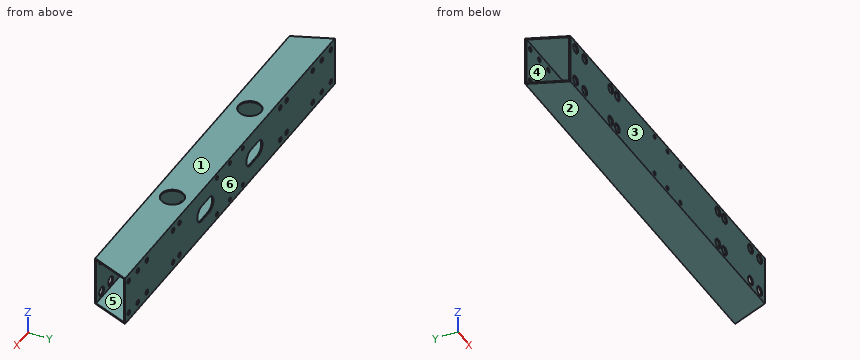
```python
from build123d import *

# Parameters (mm, degrees)
SKETCH_1_W          = 40
SKETCH_1_H          = 30
SKETCH_1_W_2        = 38
SKETCH_1_H_2        = 28
EXTRUDE_1_DEPTH     = 325
SKETCH_2_R          = 2.025
CUT_EXTRUDE_1_DEPTH = 31
SKETCH_3_R          = 2.025
CUT_EXTRUDE_2_DEPTH = 31
SKETCH_4_R          = 1.6
CUT_EXTRUDE_3_DEPTH = 31
CUT_EXTRUDE_4_DEPTH = 41
CUT_EXTRUDE_5_REACH = 32
SKETCH_6_R          = 3.75
CUT_EXTRUDE_6_REACH = 32
SKETCH_7_R          = 3.75
CUT_EXTRUDE_7_REACH = 42
SKETCH_8_R          = 9
CUT_EXTRUDE_8_REACH = 32


with BuildPart() as part:
    # 草图1 → 凸台-拉伸1 (new body)
    with BuildSketch(Plane(origin=(0, 0, 0), x_dir=(0, 0, -1), z_dir=(1, 0, 0))):
        Rectangle(SKETCH_1_W, SKETCH_1_H)
        Rectangle(SKETCH_1_W_2, SKETCH_1_H_2, mode=Mode.SUBTRACT)
    extrude(amount=EXTRUDE_1_DEPTH)

    # 草图2 → 切除-拉伸1 (cut, through all)
    with BuildSketch(Plane.XZ.offset(15)):
        with Locations((74.5, 14)):
            Circle(SKETCH_2_R)
        with Locations((84.5, 14)):
            Circle(SKETCH_2_R)
        with Locations((84.5, -14)):
            Circle(SKETCH_2_R)
        with Locations((74.5, -14)):
            Circle(SKETCH_2_R)
        with Locations((250.5, -14)):
            Circle(SKETCH_2_R)
        with Locations((240.5, -14)):
            Circle(SKETCH_2_R)
        with Locations((240.5, 14)):
            Circle(SKETCH_2_R)
        with Locations((250.5, 14)):
            Circle(SKETCH_2_R)
    extrude(amount=-CUT_EXTRUDE_1_DEPTH, mode=Mode.SUBTRACT)

    # 草图3 → 切除-拉伸2 (cut, through all)
    with BuildSketch(Plane.XZ.offset(15)):
        with Locations((291, 14)):
            Circle(SKETCH_3_R)
        with Locations((305, 14)):
            Circle(SKETCH_3_R)
        with Locations((319, 14)):
            Circle(SKETCH_3_R)
        with Locations((319, -14)):
            Circle(SKETCH_3_R)
        with Locations((305, -14)):
            Circle(SKETCH_3_R)
        with Locations((291, -14)):
            Circle(SKETCH_3_R)
        with Locations((34, -14)):
            Circle(SKETCH_3_R)
        with Locations((20, -14)):
            Circle(SKETCH_3_R)
        with Locations((6, -14)):
            Circle(SKETCH_3_R)
        with Locations((6, 14)):
            Circle(SKETCH_3_R)
        with Locations((20, 14)):
            Circle(SKETCH_3_R)
        with Locations((34, 14)):
            Circle(SKETCH_3_R)
    extrude(amount=-CUT_EXTRUDE_2_DEPTH, mode=Mode.SUBTRACT)

    # 草图4 → 切除-拉伸3 (cut, through all)
    with BuildSketch(Plane.XZ.offset(15)):
        with Locations((142.5, 16)):
            Circle(SKETCH_4_R)
        with Locations((162.5, 16)):
            Circle(SKETCH_4_R)
        with Locations((182.5, 16)):
            Circle(SKETCH_4_R)
        with Locations((182.5, -16)):
            Circle(SKETCH_4_R)
        with Locations((162.5, -16)):
            Circle(SKETCH_4_R)
        with Locations((142.5, -16)):
            Circle(SKETCH_4_R)
    extrude(amount=-CUT_EXTRUDE_3_DEPTH, mode=Mode.SUBTRACT)

    # 草图5 → 切除-拉伸4 (cut, through all)
    with BuildSketch(Plane.XY.offset(20)):
        Polygon((0, 15), (12, -15), (0, -15), align=None)
        Polygon((313, -15), (325, -15), (325, 15), align=None)
    extrude(amount=-CUT_EXTRUDE_4_DEPTH, mode=Mode.SUBTRACT)

    # 草图6 → 切除-拉伸5 (cut, up to next)
    with BuildSketch(Plane.XZ.offset(15), mode=Mode.PRIVATE) as cut_extrude_5_sk1:
        with Locations((74.5, 14)):
            Circle(SKETCH_6_R)
    cut_extrude_5_tool1 = extrude(cut_extrude_5_sk1.sketch, amount=-CUT_EXTRUDE_5_REACH, mode=Mode.PRIVATE) & part.part
    add(cut_extrude_5_tool1.solids().sort_by_distance((74.5, -15, 14))[0], mode=Mode.SUBTRACT)
    # 草图6 → 切除-拉伸5 (cut, up to next)
    with BuildSketch(Plane.XZ.offset(15), mode=Mode.PRIVATE) as cut_extrude_5_sk2:
        with Locations((84.5, 14)):
            Circle(SKETCH_6_R)
    cut_extrude_5_tool2 = extrude(cut_extrude_5_sk2.sketch, amount=-CUT_EXTRUDE_5_REACH, mode=Mode.PRIVATE) & part.part
    add(cut_extrude_5_tool2.solids().sort_by_distance((84.5, -15, 14))[0], mode=Mode.SUBTRACT)
    # 草图6 → 切除-拉伸5 (cut, up to next)
    with BuildSketch(Plane.XZ.offset(15), mode=Mode.PRIVATE) as cut_extrude_5_sk3:
        with Locations((84.5, -14)):
            Circle(SKETCH_6_R)
    cut_extrude_5_tool3 = extrude(cut_extrude_5_sk3.sketch, amount=-CUT_EXTRUDE_5_REACH, mode=Mode.PRIVATE) & part.part
    add(cut_extrude_5_tool3.solids().sort_by_distance((84.5, -15, -14))[0], mode=Mode.SUBTRACT)
    # 草图6 → 切除-拉伸5 (cut, up to next)
    with BuildSketch(Plane.XZ.offset(15), mode=Mode.PRIVATE) as cut_extrude_5_sk4:
        with Locations((74.5, -14)):
            Circle(SKETCH_6_R)
    cut_extrude_5_tool4 = extrude(cut_extrude_5_sk4.sketch, amount=-CUT_EXTRUDE_5_REACH, mode=Mode.PRIVATE) & part.part
    add(cut_extrude_5_tool4.solids().sort_by_distance((74.5, -15, -14))[0], mode=Mode.SUBTRACT)
    # 草图6 → 切除-拉伸5 (cut, up to next)
    with BuildSketch(Plane.XZ.offset(15), mode=Mode.PRIVATE) as cut_extrude_5_sk5:
        with Locations((250.5, -14)):
            Circle(SKETCH_6_R)
    cut_extrude_5_tool5 = extrude(cut_extrude_5_sk5.sketch, amount=-CUT_EXTRUDE_5_REACH, mode=Mode.PRIVATE) & part.part
    add(cut_extrude_5_tool5.solids().sort_by_distance((250.5, -15, -14))[0], mode=Mode.SUBTRACT)
    # 草图6 → 切除-拉伸5 (cut, up to next)
    with BuildSketch(Plane.XZ.offset(15), mode=Mode.PRIVATE) as cut_extrude_5_sk6:
        with Locations((240.5, -14)):
            Circle(SKETCH_6_R)
    cut_extrude_5_tool6 = extrude(cut_extrude_5_sk6.sketch, amount=-CUT_EXTRUDE_5_REACH, mode=Mode.PRIVATE) & part.part
    add(cut_extrude_5_tool6.solids().sort_by_distance((240.5, -15, -14))[0], mode=Mode.SUBTRACT)
    # 草图6 → 切除-拉伸5 (cut, up to next)
    with BuildSketch(Plane.XZ.offset(15), mode=Mode.PRIVATE) as cut_extrude_5_sk7:
        with Locations((240.5, 14)):
            Circle(SKETCH_6_R)
    cut_extrude_5_tool7 = extrude(cut_extrude_5_sk7.sketch, amount=-CUT_EXTRUDE_5_REACH, mode=Mode.PRIVATE) & part.part
    add(cut_extrude_5_tool7.solids().sort_by_distance((240.5, -15, 14))[0], mode=Mode.SUBTRACT)
    # 草图6 → 切除-拉伸5 (cut, up to next)
    with BuildSketch(Plane.XZ.offset(15), mode=Mode.PRIVATE) as cut_extrude_5_sk8:
        with Locations((250.5, 14)):
            Circle(SKETCH_6_R)
    cut_extrude_5_tool8 = extrude(cut_extrude_5_sk8.sketch, amount=-CUT_EXTRUDE_5_REACH, mode=Mode.PRIVATE) & part.part
    add(cut_extrude_5_tool8.solids().sort_by_distance((250.5, -15, 14))[0], mode=Mode.SUBTRACT)

    # 草图7 → 切除-拉伸6 (cut, up to next)
    with BuildSketch(Plane.XZ.offset(15), mode=Mode.PRIVATE) as cut_extrude_6_sk1:
        with Locations((20, 14)):
            Circle(SKETCH_7_R)
    cut_extrude_6_tool1 = extrude(cut_extrude_6_sk1.sketch, amount=-CUT_EXTRUDE_6_REACH, mode=Mode.PRIVATE) & part.part
    add(cut_extrude_6_tool1.solids().sort_by_distance((20, -15, 14))[0], mode=Mode.SUBTRACT)
    # 草图7 → 切除-拉伸6 (cut, up to next)
    with BuildSketch(Plane.XZ.offset(15), mode=Mode.PRIVATE) as cut_extrude_6_sk2:
        with Locations((34, 14)):
            Circle(SKETCH_7_R)
    cut_extrude_6_tool2 = extrude(cut_extrude_6_sk2.sketch, amount=-CUT_EXTRUDE_6_REACH, mode=Mode.PRIVATE) & part.part
    add(cut_extrude_6_tool2.solids().sort_by_distance((34, -15, 14))[0], mode=Mode.SUBTRACT)
    # 草图7 → 切除-拉伸6 (cut, up to next)
    with BuildSketch(Plane.XZ.offset(15), mode=Mode.PRIVATE) as cut_extrude_6_sk3:
        with Locations((34, -14)):
            Circle(SKETCH_7_R)
    cut_extrude_6_tool3 = extrude(cut_extrude_6_sk3.sketch, amount=-CUT_EXTRUDE_6_REACH, mode=Mode.PRIVATE) & part.part
    add(cut_extrude_6_tool3.solids().sort_by_distance((34, -15, -14))[0], mode=Mode.SUBTRACT)
    # 草图7 → 切除-拉伸6 (cut, up to next)
    with BuildSketch(Plane.XZ.offset(15), mode=Mode.PRIVATE) as cut_extrude_6_sk4:
        with Locations((20, -14)):
            Circle(SKETCH_7_R)
    cut_extrude_6_tool4 = extrude(cut_extrude_6_sk4.sketch, amount=-CUT_EXTRUDE_6_REACH, mode=Mode.PRIVATE) & part.part
    add(cut_extrude_6_tool4.solids().sort_by_distance((20, -15, -14))[0], mode=Mode.SUBTRACT)
    # 草图7 → 切除-拉伸6 (cut, up to next)
    with BuildSketch(Plane.XZ.offset(15), mode=Mode.PRIVATE) as cut_extrude_6_sk5:
        with Locations((305, -14)):
            Circle(SKETCH_7_R)
    cut_extrude_6_tool5 = extrude(cut_extrude_6_sk5.sketch, amount=-CUT_EXTRUDE_6_REACH, mode=Mode.PRIVATE) & part.part
    add(cut_extrude_6_tool5.solids().sort_by_distance((305, -15, -14))[0], mode=Mode.SUBTRACT)
    # 草图7 → 切除-拉伸6 (cut, up to next)
    with BuildSketch(Plane.XZ.offset(15), mode=Mode.PRIVATE) as cut_extrude_6_sk6:
        with Locations((291, -14)):
            Circle(SKETCH_7_R)
    cut_extrude_6_tool6 = extrude(cut_extrude_6_sk6.sketch, amount=-CUT_EXTRUDE_6_REACH, mode=Mode.PRIVATE) & part.part
    add(cut_extrude_6_tool6.solids().sort_by_distance((291, -15, -14))[0], mode=Mode.SUBTRACT)
    # 草图7 → 切除-拉伸6 (cut, up to next)
    with BuildSketch(Plane.XZ.offset(15), mode=Mode.PRIVATE) as cut_extrude_6_sk7:
        with Locations((291, 14)):
            Circle(SKETCH_7_R)
    cut_extrude_6_tool7 = extrude(cut_extrude_6_sk7.sketch, amount=-CUT_EXTRUDE_6_REACH, mode=Mode.PRIVATE) & part.part
    add(cut_extrude_6_tool7.solids().sort_by_distance((291, -15, 14))[0], mode=Mode.SUBTRACT)
    # 草图7 → 切除-拉伸6 (cut, up to next)
    with BuildSketch(Plane.XZ.offset(15), mode=Mode.PRIVATE) as cut_extrude_6_sk8:
        with Locations((305, 14)):
            Circle(SKETCH_7_R)
    cut_extrude_6_tool8 = extrude(cut_extrude_6_sk8.sketch, amount=-CUT_EXTRUDE_6_REACH, mode=Mode.PRIVATE) & part.part
    add(cut_extrude_6_tool8.solids().sort_by_distance((305, -15, 14))[0], mode=Mode.SUBTRACT)

    # 草图8 → 切除-拉伸7 (cut, up to next)
    with BuildSketch(Plane.XY.offset(20), mode=Mode.PRIVATE) as cut_extrude_7_sk1:
        with Locations((102.5, 0)):
            Circle(SKETCH_8_R)
    cut_extrude_7_tool1 = extrude(cut_extrude_7_sk1.sketch, amount=-CUT_EXTRUDE_7_REACH, mode=Mode.PRIVATE) & part.part
    add(cut_extrude_7_tool1.solids().sort_by_distance((102.5, 0, 20))[0], mode=Mode.SUBTRACT)
    # 草图8 → 切除-拉伸7 (cut, up to next)
    with BuildSketch(Plane.XY.offset(20), mode=Mode.PRIVATE) as cut_extrude_7_sk2:
        with Locations((222.5, 0)):
            Circle(SKETCH_8_R)
    cut_extrude_7_tool2 = extrude(cut_extrude_7_sk2.sketch, amount=-CUT_EXTRUDE_7_REACH, mode=Mode.PRIVATE) & part.part
    add(cut_extrude_7_tool2.solids().sort_by_distance((222.5, 0, 20))[0], mode=Mode.SUBTRACT)

    # 草图9 → 切除-拉伸8 (cut, up to next)
    with BuildSketch(Plane(origin=(0, 15, 0), x_dir=(1, 0, 0), z_dir=(0, 1, 0)), mode=Mode.PRIVATE) as cut_extrude_8_sk1:
        with BuildLine():
            Line((118.5, 6.5), (130.5, 6.5))
            ThreePointArc((130.5, 6.5), (137, 0), (130.5, -6.5))
            Line((130.5, -6.5), (118.5, -6.5))
            ThreePointArc((118.5, -6.5), (112, 0), (118.5, 6.5))
        make_face()
    cut_extrude_8_tool1 = extrude(cut_extrude_8_sk1.sketch, amount=-CUT_EXTRUDE_8_REACH, mode=Mode.PRIVATE) & part.part
    add(cut_extrude_8_tool1.solids().sort_by_distance((124.5, 15, 0))[0], mode=Mode.SUBTRACT)
    # 草图9 → 切除-拉伸8 (cut, up to next)
    with BuildSketch(Plane(origin=(0, 15, 0), x_dir=(1, 0, 0), z_dir=(0, 1, 0)), mode=Mode.PRIVATE) as cut_extrude_8_sk2:
        with BuildLine():
            Line((206.5, 6.5), (194.5, 6.5))
            ThreePointArc((194.5, 6.5), (188, 0), (194.5, -6.5))
            Line((194.5, -6.5), (206.5, -6.5))
            ThreePointArc((206.5, -6.5), (213, 0), (206.5, 6.5))
        make_face()
    cut_extrude_8_tool2 = extrude(cut_extrude_8_sk2.sketch, amount=-CUT_EXTRUDE_8_REACH, mode=Mode.PRIVATE) & part.part
    add(cut_extrude_8_tool2.solids().sort_by_distance((200.5, 15, 0))[0], mode=Mode.SUBTRACT)


solid = part.part
```
Read the model definition and answer for the solid it produces. Units are mm, in the model's axes. Face numbers are marked on the shaded views. A direction names the side the tool comes from. Coordinates: 2 decimals unless noted, no trailing zeros. Order: outer loops, then holes, each group sorted by start corner. A loop starts at its lowest first (then second) coordinate and runs counter-clockwise, first axis right, second up. Notation, with made-up numbers: (32, -8.5) - (72, -8.5) arc R22 ccw to (72, 19.5) - close; hole circle Ø10 at (-14.5, -30.5). An arc over 180 degrees is marked (long way). Answer as a JSON object with one key per item and string values. Group by question number.
Item 1: A tool of negligible diameter and unlimited length cuts with its end or side. For the marked faces 5 and 6, from which of +Z, -Z, +X, -X, +Y, -Y can it reach the whole face along a straight path? Write none if from no direction.
Item 2: A flat-ended cylindrical pin translates along its axis: P1, Ø2.5, axis at x = 240.5, z = -14, coming from the +Y side. Find the tip coordinate at first contact, or state that the pin passes through.
Item 3: Section A-A (y = 0) is taken. Give the vertices of the cut face in (x, z).
Item 4: The mould has two halves that part along Z. Classify the marked faces 1, 2, 3 and 4: +Z half, -Z half, draft (parallel to the pull), parting line (faces both ways), or undercut.
Item 5: Section B-B (x = 150) is taken. Give the vertices of the cut face in (y, z).
Item 6: Consider probe 1 along Z at (x, y) = (74.5, 14.4) (3 decimals); probe 2 along Z at (x, y) = (244.5, 2); probe 3 along Y at (x, z) = (13.5, 2). Determine where each line is inside the solid, lowest interval first. Write a range as from..to.
Results are:
{
 "1": {"face 5": "+X, -X", "face 6": "+Z, -Z, +X, -X, +Y"},
 "2": {"P1": "passes through"},
 "3": {"outline": "(6, -20) - (319, -20) - (319, -19) - (6, -19) - close; (6, 19) - (93.5, 19) - (93.5, 20) - (6, 20) - close; (111.5, 19) - (213.5, 19) - (213.5, 20) - (111.5, 20) - close; (231.5, 19) - (319, 19) - (319, 20) - (231.5, 20) - close"},
 "4": {"face 1": "+Z half", "face 2": "-Z half", "face 3": "draft", "face 4": "undercut"},
 "5": {"outline": "(-15, -20) - (15, -20) - (15, 20) - (-15, 20) - close; hole (-14, -19) - (14, -19) - (14, 19) - (-14, 19) - close"},
 "6": {"probe 1": "z = -20..-16.025, -11.975..11.975, 16.025..20", "probe 2": "z = -20..-19, 19..20", "probe 3": "y = -15..-14, 14..15"}
}
